from build123d import *

# Parameters (mm, degrees)
SKETCH075_R             = 6.5
SKETCH075_R_2           = 2.5
PAD039_DEPTH            = 6
SKETCH076_R             = 5
SKETCH076_R_2           = 2.522437
PAD040_DEPTH            = 7
SKETCH077_R             = 6.5
SKETCH077_R_2           = 2.522437
PAD041_DEPTH            = 1
SKETCH078_R             = 1
PAD042_DEPTH            = 7
BODY025_ROLL_ANGLE      = 135
BODY025_PLACEMENT_ANGLE = 180
SKETCH082_R             = 15
PAD043_DEPTH            = 8.5
POCKET027_DEPTH         = 2.5
POLARPATTERN019_COUNT   = 4
SKETCH079_R             = 1
HOLE007_DEPTH           = 25
POLARPATTERN018_COUNT   = 4
SKETCH080_R             = 4
POCKET026_DEPTH         = 6.001
BODY026_PLACEMENT_ANGLE = 90
POCKET028_DEPTH         = 7
POLARPATTERN020_COUNT   = 2
POLARPATTERN020_ANGLE   = 90


with BuildPart() as polea006:
    # Sketch075 → Pad039 (new body)
    with BuildSketch(Plane.YZ):
        Circle(SKETCH075_R)
        Circle(SKETCH075_R_2, mode=Mode.SUBTRACT)
    extrude(amount=PAD039_DEPTH)

    # Sketch076 (on Face3 of Pad039) → Pad040 (join)
    with BuildSketch(Plane(origin=(0, 0, 0), x_dir=(0, 1, 0), z_dir=(-1, 0, 0))):
        Circle(SKETCH076_R)
        Circle(SKETCH076_R_2, mode=Mode.SUBTRACT)
    extrude(amount=PAD040_DEPTH)

    # Sketch077 (on Face6 of Pad040) → Pad041 (join)
    with BuildSketch(Plane(origin=(-7, 0, 0), x_dir=(0, 1, 0), z_dir=(-1, 0, 0))):
        Circle(SKETCH077_R)
        Circle(SKETCH077_R_2, mode=Mode.SUBTRACT)
    extrude(amount=PAD041_DEPTH)

    # Sketch078 → Pad042 (join)
    with BuildSketch(Plane.XZ):
        with Locations((3, 0)):
            Circle(SKETCH078_R)
    extrude(amount=PAD042_DEPTH)


with BuildPart() as polea006_1:
    # Body025 roll: moved
    add(polea006.part.rotate(Axis((0, 0, 0), (1, 0, 0)), BODY025_ROLL_ANGLE))


with BuildPart() as polea006_2:
    # Body025 placement: moved
    add(polea006_1.part.rotate(Axis((0, 0, 0), (0, 0, 1)), BODY025_PLACEMENT_ANGLE))


with BuildPart() as body027:
    # Sketch082 → Pad043 (new body)
    with BuildSketch(Plane.XY):
        Circle(SKETCH082_R)
    extrude(amount=PAD043_DEPTH)

    # Sketch081 (on Face3 of Pad043) → Pocket027 (cut)
    with BuildSketch(Plane.XY.offset(8.5)):
        with BuildLine():
            ThreePointArc((-5.26869, 1.578261), (0, -5.5), (5.26869, 1.578261))
            Line((2.107476, 12.131304), (5.26869, 1.578261))
            ThreePointArc((2.107476, 12.131304), (0, 13.7), (-2.107476, 12.131304))
            Line((-2.107476, 12.131304), (-5.26869, 1.578261))
        make_face()
    pocket027 = extrude(amount=-POCKET027_DEPTH, mode=Mode.SUBTRACT)

    # PolarPattern019: Pocket027 ×4 about axis
    polarpattern019_axis = Axis((0, 0, 8.5), (0, 0, 1))
    for i in range(1, POLARPATTERN019_COUNT):
        add(pocket027.rotate(polarpattern019_axis, i * 360 / POLARPATTERN019_COUNT), mode=Mode.SUBTRACT)

    # Sketch079 (on Face21 of PolarPattern019) → Hole007 (cut)
    with BuildSketch(Plane.XY.offset(6)):
        with Locations((0, 11)):
            Circle(SKETCH079_R)
    hole007 = extrude(amount=-HOLE007_DEPTH, mode=Mode.SUBTRACT)

    # PolarPattern018: Hole007 ×4 about axis
    polarpattern018_axis = Axis((0, 0, 6), (0, 0, 1))
    for i in range(1, POLARPATTERN018_COUNT):
        add(hole007.rotate(polarpattern018_axis, i * 360 / POLARPATTERN018_COUNT), mode=Mode.SUBTRACT)

    # Sketch080 (on Face25 of PolarPattern018) → Pocket026 (cut, through all)
    with BuildSketch(Plane.XY.offset(6)):
        Circle(SKETCH080_R)
    extrude(amount=-POCKET026_DEPTH, mode=Mode.SUBTRACT)


with BuildPart() as body027_1:
    # Body026 placement: moved
    add(body027.part.moved(Location((0, 0, 0))).rotate(Axis((0, 0, 0), (0, -1, 0)), BODY026_PLACEMENT_ANGLE))

    # Cut004: cut polea006
    add(polea006_2.part, mode=Mode.SUBTRACT)

    # Sketch083 (on Face3 of BaseFeature004) → Pocket028 (cut)
    with BuildSketch(Plane(origin=(-8.5, 0, 0), x_dir=(0, -1, 0), z_dir=(-1, 0, 0))):
        Polygon((2.474874, -4.596194), (4.596194, -2.474874), (12.374369, -10.253048), (10.253048, -12.374369), align=None)
    pocket028 = extrude(amount=-POCKET028_DEPTH, mode=Mode.SUBTRACT)

    # PolarPattern020: Pocket028 ×2 about axis
    polarpattern020_axis = Axis((-8.5, 0, 0), (-1, 0, 0))
    for i in range(1, POLARPATTERN020_COUNT):
        add(pocket028.rotate(polarpattern020_axis, i * POLARPATTERN020_ANGLE / (POLARPATTERN020_COUNT - 1)), mode=Mode.SUBTRACT)


solid = body027_1.part
CAD build for the part. Positions are in the model's coordinates, mm. A direction names the side the tool comes from. Round coordinates to 2 decimals unless told otherwise and drop trailing zeros. Loops run counter-clockwise (first coordinate to the right, second up) from the corner with the lowest first, then second, coordinate; pieces in that order, holes last.
(1) Wall check: line 1 along Y through (x, z) = (-3.2, 0); line 2 along X through (y, z) = (-9.75, -11). Give the ranges that are in metal, low to high.
(2) Two-plate mould, pull along Z, no slides. Class faces 1 (the flat face through (-8.5, 8, -4)), 2 (the cylindrical face through (-4.191, 0.66, -14.985)), 3 (the flat face through (-5.049, -8.616, 6.495)): +Z half, -Z half, draft (parallel to the pull), parting line (faces both ways), or undercut.
(3) Cut at A-A (x = -6.75). Give the cut face in (y, z), plus the area to 3 significant figures.
(4) Which spindle directions (+Z, -Z, +X, -X, +Y, -Y) get a long thin tool onto all of the face, cutting with end or side? Do faces 4 (the cylindrical face through (-3, 0, 10)), 5 (the flat face through (-6, -9.6, 0.1)). Say none if no direction does.
(5) Cut at B-B (y = 0). Give the cut face in (x, z), plus the area to 3 significant figures.
(6) Drop flat-ended pins along their axis: pin 1 (2.5 mm diameter, centred on y = -0.5, z = 10.5, fed in from -X); pin 2 (3 mm diameter, centred on x = -4.5, y = 6, fed in from +Z); pin 3 (1.5 mm diameter, centred on x = -5, z = 4, fed in from +Y); pin 4 (1.8 mm diameter, centred on y = 0, z = 11, fed in from +X). Give the stop position or say it passes through.
(7) Cut at D-D (z = 11). Give the cut face in (x, y), plus the area to 3 significant figures.
Findings below:
1. line 1: y = -15 to -12, -10 to -6.5, 6.5 to 10, 12 to 15
1. line 2: x = -1.5 to 0
2. face 1: draft
2. face 2: parting line
2. face 3: undercut
3. outline: (-12.13, -2.11) arc R2.2 cw to (-12.13, 2.11) - (-6.05, 3.93) - (-11.61, 9.49) arc R15 ccw to (-11.61, -9.49) - (-6.05, -3.93) - close; (-9.49, -11.61) arc R15 ccw (long way) to (-9.49, 11.61) - (-3.93, 6.05) - (-2.11, 12.13) arc R2.2 cw to (2.11, 12.13) - (4.42, 4.42) - (12.13, 2.11) arc R2.2 cw to (12.13, -2.11) - (4.42, -4.42) - (2.11, -12.13) arc R2.2 cw to (-2.11, -12.13) - (-3.93, -6.05) - close
3. area: 358 mm2
4. face 4: +X, -X
4. face 5: -X
5. outline: (-8.5, -15) - (0, -15) - (0, -12) - (-6, -12) - (-6, -13.7) - (-8.5, -13.7) - close; (-8.5, 13.7) - (-6, 13.7) - (-6, 12) - (0, 12) - (0, 15) - (-8.5, 15) - close; (-6, -10) - (0, -10) - (0, -6.5) - (-6, -6.5) - close; (-6, 6.5) - (0, 6.5) - (0, 10) - (-6, 10) - close
5. area: 84.5 mm2
6. pin 1: stops at x = -6
6. pin 2: stops at z = 14.31
6. pin 3: stops at y = 14.64
6. pin 4: passes through
7. outline: (-8.5, -8.88) - (-1.5, -8.88) - (-1.5, -10.2) - (0, -10.2) - (0, -1) - (-6, -1) - (-6, -2.45) - (-8.5, -2.45) - close; (-8.5, 2.45) - (-6, 2.45) - (-6, 1) - (0, 1) - (0, 10.2) - (-8.5, 10.2) - close
7. area: 140 mm2
